Study the drawing (mm; zero at the part's minimum x, y, z) and answer. Round coordinates to 2 decimals unless told otherwise and drop trailing zeros. Write each loop counter-clockwise with the first axis right and the second up, starting at its lowest first coordinate (ties: lowest second). Pieces come first, ordered by that corner, then holes.
(1) A cutting plane is placed at D-D, the plane z = 3.55. Give the vertices of the cut face in (x, y), and give its area (3 significant figures).
(2) The mould has two halves that part along X. Classify the marked faces 1, 2 and 3: +X half, -X half, draft (parallel to the pull), parting line (faces both ways), or undercut.
(3) Each of these flat-tipped pins is pushed along its axis until it touches: pin 1 Ø10 at (x, y) = (37.5, 10) entering from -Z; pin 2 Ø1 at (x, z) = (10, 4.5) entering from -Y; pin 3 Ø1 at (y, z) = (18.5, 1) entering from +X; pin 4 Ø2 at (y, z) = (17.5, 5) entering from +X. Where does it stop, or does it pass through?
(4) Find the intervals of material crossed by probe 1 along Y at (x, z) = (27, 1.3); probe 2 along X at (y, z) = (16, 3.9); probe 3 along X at (y, z) = (26.5, 2.35) (1 decimal), in increasing order.
(5) A cutting plane is placed at A-A, the plane x = 27. Give the vertices of the cut face in (y, z).
(6) A cutting plane is placed at C-C, the plane x = 12. Give the vertices of the cut face in (y, z).
(7) A cutting plane is placed at B-B, the plane y = 4. Give the vertices of the cut face in (x, z), and give its area (3 significant figures).
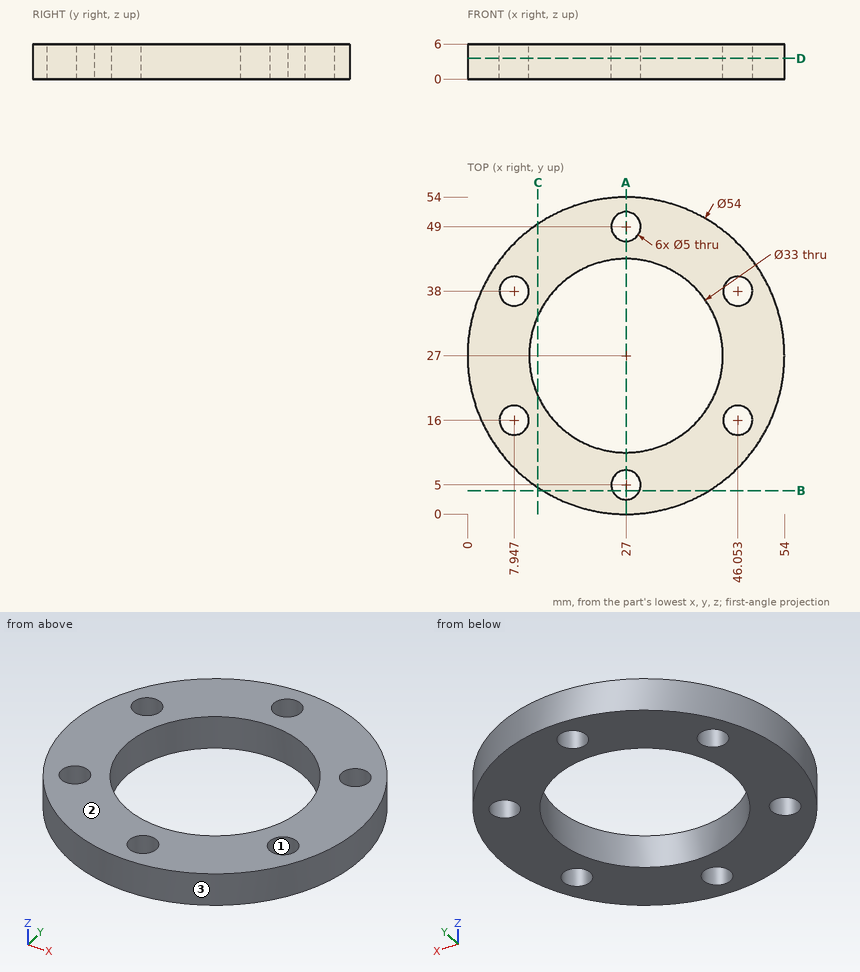
Solutions:
1. outline: circle Ø54 at (27, 27); hole circle Ø5 at (7.95, 16); hole circle Ø5 at (7.95, 38); hole circle Ø33 at (27, 27); hole circle Ø5 at (27, 5); hole circle Ø5 at (27, 49); hole circle Ø5 at (46.05, 16); hole circle Ø5 at (46.05, 38)
1. area: 1,320 mm2
2. face 1: undercut
2. face 2: draft
2. face 3: parting line
3. pin 1: stops at z = 0
3. pin 2: stops at y = 5.63
3. pin 3: stops at x = 52.79
3. pin 4: stops at x = 52.63
4. probe 1: y = 0 to 2.5, 7.5 to 10.5, 43.5 to 46.5, 51.5 to 54
4. probe 2: x = 2.34 to 5.45, 10.45 to 14.7, 39.3 to 43.55, 48.55 to 51.66
4. probe 3: x = 0 to 10.5, 43.5 to 54
5. outline: (0, 0) - (2.5, 0) - (2.5, 6) - (0, 6) - close; (7.5, 0) - (10.5, 0) - (10.5, 6) - (7.5, 6) - close; (43.5, 0) - (46.5, 0) - (46.5, 6) - (43.5, 6) - close; (51.5, 0) - (54, 0) - (54, 6) - (51.5, 6) - close
6. outline: (4.55, 0) - (20.13, 0) - (20.13, 6) - (4.55, 6) - close; (33.87, 0) - (49.45, 0) - (49.45, 6) - (33.87, 6) - close
7. outline: (12.86, 0) - (24.71, 0) - (24.71, 6) - (12.86, 6) - close; (29.29, 0) - (41.14, 0) - (41.14, 6) - (29.29, 6) - close
7. area: 142 mm2
